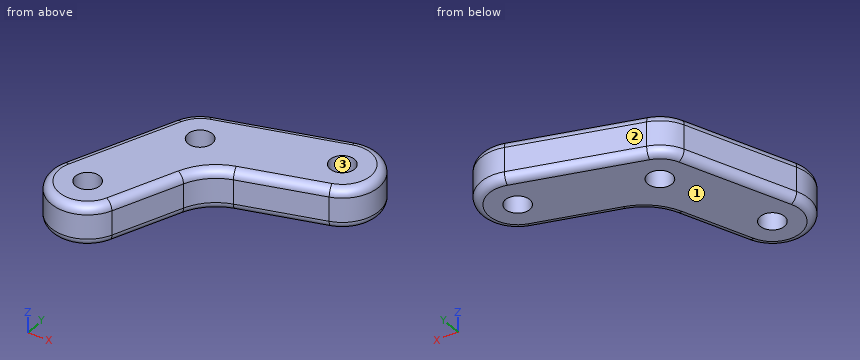
Autodesk Inventor part; units mm, degrees
ref_plane "YZ Plane" through (0, 0, 0) normal (1, 0, 0) x (0, 1, 0)
ref_plane "XZ Plane" through (0, 0, 0) normal (0, 1, 0) x (-1, 0, 0)
ref_plane "XY Plane" through (0, 0, 0) normal (0, 0, 1) x (1, 0, 0)
sketch "Sketch1" plane through (0, 0, 0) normal (0, 0, 1) x (1, 0, 0)
  circle A0 centre (2.1561, 2.8874) radius 18
  circle A1 centre (80.1561, 70.6294) radius 18
  circle A2 centre (22.8814, 52.7519) radius 18
  line L0 (74.7929, 87.8119) -> (17.5182, 69.9343)
  line L1 (-14.4653, 9.7959) -> (6.2599, 59.6603)
  line L2 (18.7776, -4.021) -> (39.5029, 45.8434)
  line L3 (85.5194, 53.447) -> (28.2447, 35.5695)
  circle A3 centre (2.1561, 2.8874) radius 6
  circle A4 centre (22.8814, 52.7519) radius 6
  circle A5 centre (80.1561, 70.6294) radius 6
  point P0 (0, 0)
  point P1 (36.2744, 38.0758)
  dimension "d0" = 36
  dimension "d1" = 36
  dimension "d2" = 54
  dimension "d3" = 60
  dimension "d6" = 12
extrude "Extrusion1" add sketch "Sketch1" along normal blind 20
fillet "Fillet2" radius 24 1 edges at (36.2744, 38.0758, 10)
fillet "Fillet1" radius 4 14 edges at (10.748, 66.0477, 20) (-4.1027, 34.7281, 20) (-4.7523, -13.734, 20) (25.3737, 11.849, 20) (97.3386, 75.9927, 20) (66.2501, 47.4324, 20) (46.1555, 78.8731, 20) (10.748, 66.0477, 0) (-4.1027, 34.7281, 0) (-4.7523, -13.734, 0) (25.3737, 11.849, 0) (97.3386, 75.9927, 0) (66.2501, 47.4324, 0) (46.1555, 78.8731, 0)
properties part number "SteelPost"
Geometry: final body of the model. Coordinates: model frame, mm. Face numbers are marked on the shaded views. Give positions to 0.01 mm unless a question says otherwise; leave off trailing zeros. Order: outer loops, then holes, each group sorted by start corner. A loop starts at its lowest first (then second) coordinate and runs counter-clockwise, first axis right, second up. Notation, with made-up numbers: (-20, -1.5) -> (35, -1.5) arc R11 ccw to (35, 4.5) -> close; hole circle Ø8 at (4, 84). An arc over 180 degrees is marked (long way). Put each result on its own line as item: value.
Q1. Draft query along Y for the marked faces 1, 2 and 3. Return one class per face: released by +Y, released by -Y, zero draft, split by the parting line, or undercut.
Here are the results:
face 1: zero draft
face 2: released by +Y
face 3: undercut
Q2. Section A-A, the plane z = 12. Return loops of the section in (x, y).
Here are the results:
outline: (-14.47, 9.8) arc R18 ccw to (18.78, -4.02) -> (31.97, 27.72) arc R24 cw to (46.98, 41.42) -> (85.52, 53.45) arc R18 ccw to (74.79, 87.81) -> (17.52, 69.93) arc R18 ccw to (6.26, 59.66) -> close; hole circle Ø12 at (2.16, 2.89); hole circle Ø12 at (22.88, 52.75); hole circle Ø12 at (80.16, 70.63)
Q3. Pin query (flat end, axial travel): pin 1 (14 mm diameter, centred on x = 2.16, y = 2.89, fed in from +Z); pin 2 (9.5 mm diameter, centred on x = 80.16, y = 70.63, fed in from -Z); pin 3 (8 mm diameter, centred on y = 28, z = 17, fed in from +X); pin 4 (2 mm diameter, centred on x = 10, z = 3.5, fed in from +Y). Return the tip coordinate at first contact, or that it passes through.
Here are the results:
pin 1: stops at z = 20
pin 2: passes through
pin 3: stops at x = 34.23
pin 4: stops at y = 66.24
Q4. Section B-B, the plane z = 1.5. Return loops of the section in (x, y) (1 decimal).
Here are the results:
outline: (-13.7, 9.5) arc R17.1 ccw to (18, -3.7) -> (31.2, 28.1) arc R24.9 cw to (46.7, 42.3) -> (85.3, 54.3) arc R17.1 ccw to (75.1, 87) -> (17.8, 69.1) arc R17.1 ccw to (7.1, 59.3) -> close; hole circle Ø12 at (2.2, 2.9); hole circle Ø12 at (22.9, 52.8); hole circle Ø12 at (80.2, 70.6)
Q5. Material intervals for L1, parallel to Y at x = 77, z = 7.75; L2, parallel to X at y = 3, z = 18.25; L3, parallel to Y at x = -1, z = 8, sorted ascending.
Here are the results:
L1: y = 50.79 to 65.53, 75.73 to 88.35
L2: x = -15.15 to -3.84, 8.16 to 20.95
L3: y = -14.83 to -2.22, 7.99 to 42.19
